Check sheet for the drawn part. Datum: minimum x, y, z corner. Units: mm. Coordinates: 2 decimals unless noted, no trailing zeros. Loops run counter-clockwise (first coordinate to the right, second up) from the corner with the lowest first, then second, coordinate; pieces in that order, holes last.
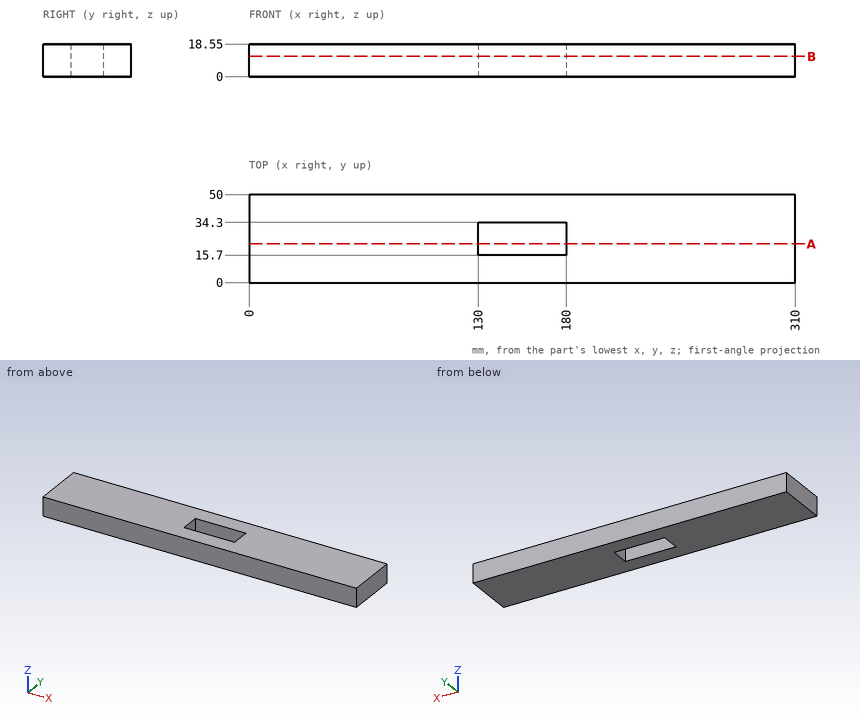
1) Section check B-B on z = 11.5. Enter the section's corners in (x, y), plus the area to 3 significant figures.
Answer sheet:
outline: (0, 0) - (310, 0) - (310, 50) - (0, 50) - close; hole (130, 15.7) - (180, 15.7) - (180, 34.3) - (130, 34.3) - close
area: 14,600 mm2
2) Section check A-A on y = 22. Enter the section's corners in (x, z).
Answer sheet:
outline: (0, 0) - (130, 0) - (130, 18.55) - (0, 18.55) - close; (180, 0) - (310, 0) - (310, 18.55) - (180, 18.55) - close
3) Scan lines: line 1 (X direction, y = 21, z = 11.5); line 2 (Y direction, x = 152.5, z = 17). Record each from-to range of solid material in increasing order.
Answer sheet:
line 1: x = 0 to 130, 180 to 310
line 2: y = 0 to 15.7, 34.3 to 50
